For this review, take the finished solid that the model builds, in its own axes (mm). A direction names the side the tool comes from. Coordinates: 2 decimals unless noted, no trailing zeros. Write each loop counter-clockwise with the first axis right and the second up, starting at its lowest first coordinate (ties: lowest second). Pieces come first, ordered by that corner, then holes. Notation, with made-up numbers: (54, -13.5) -> (102, -13.5) arc R16 ccw to (102, 4.5) -> close; hole circle Ø2 at (-24.5, 88.25). An arc over 180 degrees is marked (long way). Put each result on its own line as item: value. Start each with the question number.
Item 1: For faces 4 (the cylindrical face through (14.456, -5.586, 29.033)), 5 (the cylindrical face through (14.577, -3.16, 7.65)), 6 (the cylindrical face through (-13.78, -5.586, 28.773)), 7 (the cylindrical face through (-0.66, -3.16, -16.45)), 8 (the cylindrical face through (-14, -1, 29)), list the 3-axis set-ups (+Z, -Z, +X, -X, +Y, -Y) from which the entire face can be reached by the end or side of a thin tool; tool diameter is ignored.
Item 2: Insertion check: P1, Ø1.5, axis at x = 34.5, y = -1.5, coming from the -Z side; P2, Ø1.5, axis at y = -1, z = -25.5, coming from the -X side; P3, Ø24, axis at x = 47.73, z = -27.56, coming from the +Y side. Each pin has a flat end and moves straight along its axis. Give the tip position at first contact, or say it passes through.
Item 3: The part is to be moulded in two halves that separate along Z. For faces 1 (the cylindrical face through (40.085, -3.131, -20.545)), 2 (the cylindrical face through (-62.58, -3.13, -35.88)), 3 (the flat face through (0, -6.35, -12)), say which applies: +Z half, -Z half, draft (parallel to the pull), parting line (faces both ways), or undercut.
Item 4: To check wall thickness, follow L1, parallel to Z at x = 0, y = -1.75; L2, parallel to X at y = -1.5, z = -35.5; L3, parallel to X at y = -1, z = -20. State the ranges of each line that lie inside material, in increasing order.
Item 5: Consider section A-A on x = 54.5. Give the boundary of the cut face in (y, z).
Item 6: Consider section B-B on y = -5. Give the boundary of the cut face in (x, z), and give its area (3 significant figures).
```python
from build123d import *

# Parameters (mm, degrees)
F0_R     = 10.3857806341
F0_R_2   = 10.3786468128
F1_DEPTH = 6.35
F2_R     = 2.54
F3_R     = 2.54


with BuildPart() as f1:
    # F0 (on Front) → F1 (new body)
    with BuildSketch(Plane.XZ):
        with BuildLine():
            Line((14.3325142405, 8.0979142801), (16.0034097486, 49.3313107205))
            ThreePointArc((16.0034097486, 49.3313107205), (-0.4850827816, 72.1303829543), (-15.6475718809, 48.4287584328))
            Line((-15.6475718809, 48.4287584328), (-13.390063044, 9.576188794))
            ThreePointArc((-13.390063044, 9.576188794), (-13.7979919658, 8.9784518628), (-14.1792566045, 8.3633642923))
            ThreePointArc((-14.1792566045, 8.3633642923), (-14.6745633827, -7.4601856322), (-1.598191245, -16.3842291514))
            ThreePointArc((-1.598191245, -16.3842291514), (-0.876571417, -16.438637495), (-0.153257636, -16.4612785724))
            ThreePointArc((-0.153257636, -16.4612785724), (13.7979919658, -8.9784518628), (14.988254289, 6.8080403574))
            ThreePointArc((14.988254289, 6.8080403574), (14.6745633827, 7.4601856322), (14.3325142405, 8.0979142801))
        make_face()
        Circle(F0_R, mode=Mode.SUBTRACT)
        with Locations((0, 55.1193505526)):
            Circle(F0_R_2, mode=Mode.SUBTRACT)
        with BuildLine():
            Line((49.764321017, -10.66318446), (14.988254289, 6.8080403574))
            ThreePointArc((14.988254289, 6.8080403574), (13.7979919658, -8.9784518628), (-0.153257636, -16.4612785724))
            Line((-0.153257636, -16.4612785724), (34.7204634116, -38.5250147497))
            ThreePointArc((34.7204634116, -38.5250147497), (62.709285414, -35.6450974653), (49.764321017, -10.66318446))
        make_face()
        with Locations((47.7347578186, -27.5596752763)):
            Circle(F0_R_2, mode=Mode.SUBTRACT)
        with BuildLine():
            ThreePointArc((-1.598191245, -16.3842291514), (-14.6745633827, -7.4601856322), (-14.1792566045, 8.3633642923))
            Line((-14.1792566045, 8.3633642923), (-50.7238731603, -10.8062959708))
            ThreePointArc((-50.7238731603, -10.8062959708), (-62.2242026323, -36.485285489), (-34.1167491361, -37.7655739728))
            Line((-34.1167491361, -37.7655739728), (-1.598191245, -16.3842291514))
        make_face()
        with Locations((-47.7347578186, -27.5596752763)):
            Circle(F0_R_2, mode=Mode.SUBTRACT)
    extrude(amount=F1_DEPTH)

    # F2
    f2_edges = [f1.edges().sort_by_distance(p)[0] for p in [
        (15.167962, 0, 28.714613),
        (-14.518817, 0, 29.002474),
        (32.376288, 0, -1.927572),
        (17.283603, 0, -27.493147),
        (-17.85747, 0, -27.074902),
        (-32.451565, 0, -1.221466),
    ]]
    fillet(f2_edges, radius=F2_R)

    # F3
    f3_edges = [f1.edges().sort_by_distance(p)[0] for p in [
        (15.167962, -6.35, 28.714613),
        (-14.518817, -6.35, 29.002474),
        (-32.451565, -6.35, -1.221466),
        (-17.85747, -6.35, -27.074902),
        (17.283603, -6.35, -27.493147),
        (32.376288, -6.35, -1.927572),
    ]]
    fillet(f3_edges, radius=F3_R)


solid = f1.part
```
Return value:
1. face 4: +X, -Y
1. face 5: +X
1. face 6: -X, -Y
1. face 7: -Z
1. face 8: -X, +Y
2. P1: z = -39.12
2. P2: x = -64.7
2. P3: y = 0
3. face 1: undercut
3. face 2: parting line
3. face 3: draft
4. L1: -16.46 to -10.39, 10.39 to 44.74, 65.5 to 72.14
4. L2: -62.79 to -54.42, -41.05 to -31.08, 30.36 to 41.05, 54.42 to 62.79
4. L3: -62.98 to -54.85, -40.62 to -8.04, 6.41 to 40.62, 54.85 to 62.98
5. outline: (-6.35, -43.18) -> (0, -43.18) -> (0, -35.43) -> (-6.35, -35.43) -> close; (-6.35, -19.69) -> (0, -19.69) -> (0, -11.94) -> (-6.35, -11.94) -> close
6. outline: (-49.83, -10.67) arc R17.02 ccw (long way) to (-33.64, -37.1) -> (-2.06, -16.33) arc R16.46 ccw to (0.39, -16.46) -> (34.16, -37.82) arc R17.02 ccw (long way) to (48.95, -10.59) -> (15.17, 6.38) arc R16.46 ccw to (14.06, 8.57) -> (15.67, 48.49) arc R17.02 ccw (long way) to (-15.31, 47.68) -> (-13.12, 9.95) arc R16.46 ccw to (-14.45, 7.89) -> close; hole circle Ø20.76 at (-47.73, -27.56); hole circle Ø20.77 at (0, 0); hole circle Ø20.76 at (0, 55.12); hole circle Ø20.76 at (47.73, -27.56)
6. area: 4,530 mm^2
